```python
from build123d import *

# Parameters (mm, degrees)
SKETCH1_R           = 1.5875
SKETCH1_R_2         = 3.96875
BOSS_EXTRUDE1_DEPTH = 3.175


with BuildPart() as part:
    # Sketch1 → Boss-Extrude1 (new body)
    with BuildSketch(Plane(origin=(0, 0, 0), x_dir=(1, 0, 0), z_dir=(0, 1, 0))):
        with BuildLine():
            Line((4.906744273, 1.778), (60.663965564, 4.700112147))
            ThreePointArc((60.663965564, 4.700112147), (62.585298916, 5.014270589), (64.392175829, 5.739124507))
            ThreePointArc((64.392175829, 5.739124507), (73.97115, 0), (64.392175829, -5.739124507))
            ThreePointArc((64.392175829, -5.739124507), (62.585298916, -5.014270589), (60.663965564, -4.700112147))
            Line((60.663965564, -4.700112147), (4.906744273, -1.778))
            ThreePointArc((4.906744273, -1.778), (3.494086568, -1.971116067), (2.251338568, -2.670024513))
            ThreePointArc((2.251338568, -2.670024513), (-3.4925, 0), (2.251338568, 2.670024513))
            ThreePointArc((2.251338568, 2.670024513), (3.494086568, 1.971116067), (4.906744273, 1.778))
        make_face()
        with Locations(Location((0, 0, 0), (0, 0, 270))):
            Circle(SKETCH1_R, mode=Mode.SUBTRACT)
        with Locations(Location((67.4624, 0, 0), (0, 0, 270))):
            Circle(SKETCH1_R_2, mode=Mode.SUBTRACT)
    extrude(amount=BOSS_EXTRUDE1_DEPTH)


solid = part.part
```
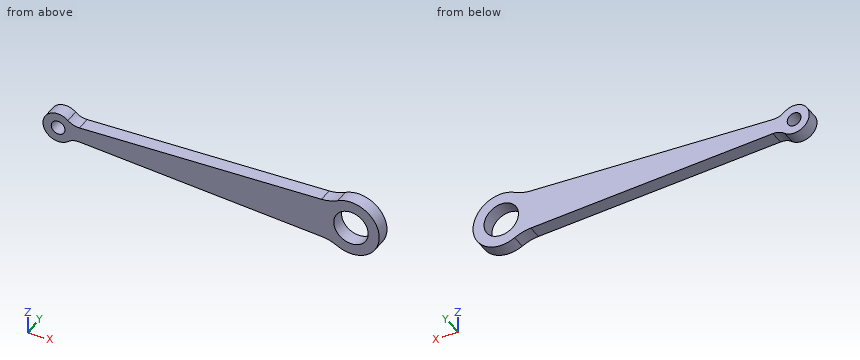
The model under review builds one solid part; all positions refer to its coordinate system, in mm. Round coordinates to 2 decimals unless told otherwise and drop trailing zeros. Loops run counter-clockwise (first coordinate to the right, second up) from the corner with the lowest first, then second, coordinate; pieces in that order, holes last. Notation, with made-up numbers: (51, 59.5) - (106, 59.5) arc R23 cw to (106, 75.5) - close; hole circle Ø10 at (8.25, 47). An arc over 180 degrees is marked (long way). Write each question's results on one line, items separated by ' | '. Start each with the question number.
Q1. Insertion check: P1, Ø1, axis at x = 49.5, y = 1.5, coming from the +Z side. The pin has a flat end and moves straight along its axis. Give the tip position at first contact, or say it passes through.
Q2. Wall thickness on line 1 along X through (y, z) = (1.8, 0.25); line 2 along Z through (x, y) = (69, 2.7); line 3 along X through (y, z) = (3, 1): over which ranges is each line inside the solid? List them lowest first. Write a range as [from, to].
Q3. Take a section at A-A on z = 0. Give the boundary of the cut face in (x, y) (1 decimal).
Q4. Take a section at B-B on x = 0. Give the boundary of the cut face in (y, z) (1 decimal).
Q5. Take a section at C-C on y = 1.15. Give the boundary of the cut face in (x, z) (1 decimal), plus the area to 3 significant figures.
Q6. Take a section at D-D on x = 21. Give the boundary of the cut face in (y, z) (3 decimals), plus the area to 3 significant figures.
Data:
1) P1: stops at z = 4.14
2) line 1: x = [-3.48, -1.57], [1.57, 63.5], [71.42, 73.97] | line 2: z = [-6.32, -3.66], [3.66, 6.32] | line 3: x = [-3.35, -1.23], [1.23, 63.62], [71.3, 73.89]
3) outline: (-3.5, 0) - (-1.6, 0) - (-1.6, 3.2) - (-3.5, 3.2) - close; (1.6, 0) - (63.5, 0) - (63.5, 3.2) - (1.6, 3.2) - close; (71.4, 0) - (74, 0) - (74, 3.2) - (71.4, 3.2) - close
4) outline: (0, -3.5) - (3.2, -3.5) - (3.2, -1.6) - (0, -1.6) - close; (0, 1.6) - (3.2, 1.6) - (3.2, 3.5) - (0, 3.5) - close
5) outline: (2.3, -2.7) arc R3.8 cw to (4.9, -1.8) - (60.7, -4.7) arc R8.9 cw to (64.4, -5.7) arc R6.5 ccw (long way) to (64.4, 5.7) arc R8.9 cw to (60.7, 4.7) - (4.9, 1.8) arc R3.8 cw to (2.3, 2.7) arc R3.5 ccw (long way) to start; hole circle Ø3.2 at (0, 0); hole circle Ø7.9 at (67.5, 0) | area: 491 mm²
6) outline: (0, -2.621) - (3.175, -2.621) - (3.175, 2.621) - (0, 2.621) - close | area: 16.6 mm²
